Build history of the part. All positions in model axes, mm. Coordinates: 2 decimals unless noted, no trailing zeros. Order: outer loops, then holes, each group sorted by start corner. A loop starts at its lowest first (then second) coordinate and runs counter-clockwise, first axis right, second up. Notation, with made-up numbers: (-14, 77) - (27, 77) arc R11 ccw to (27, 88) - close; hole circle Ø2 at (79.25, 51). An arc over 180 degrees is marked (long way). One line per item, written item: value.
Autodesk Inventor part; units mm, degrees
ref_plane "YZ Plane" through (0, 0, 0) normal (1, 0, 0) x (0, 1, 0)
ref_plane "XZ Plane" through (0, 0, 0) normal (0, 1, 0) x (-1, 0, 0)
ref_plane "XY Plane" through (0, 0, 0) normal (0, 0, 1) x (1, 0, 0)
sketch "Sketch1" plane through (0, 0, 0) normal (0, 0, 1) x (1, 0, 0)
  line L0 (568, 44.5) -> (0, 44.5)
  line L1 (68, 0) -> (78, 15)
  line L2 (78, 15) -> (490, 15)
  line L3 (490, 15) -> (500, 0)
  line L4 (0, 0) -> (68, 0)
  line L5 (500, 0) -> (568, 0)
  line L6 (0, 30) -> (68, 30)
  line L7 (68, 30) -> (68, 23.5)
  line L8 (68, 23.5) -> (0, 23.5)
  line L9 (0, 44.5) -> (0, 30)
  line L10 (0, 23.5) -> (0, 0)
  line L11 (568, 30) -> (500, 30)
  line L12 (500, 30) -> (500, 23.5)
  line L13 (500, 23.5) -> (568, 23.5)
  line L14 (568, 0) -> (568, 23.5)
  line L15 (568, 30) -> (568, 44.5)
  dimension "d3" = 6.5
  dimension "d4" = 68
  dimension "d5" = 68
  dimension "d6" = 568
  dimension "d7" = 15
  dimension "d8" = 23.5
  dimension "d9" = 14.5
  dimension "d12" = 10
  dimension "d13" = 10
  dimension "d14" = 10
  dimension "d15" = 10
extrude "Extrusion1" add sketch "Sketch1" along normal blind 6.5
sketch "Sketch2" plane through (0, 0, 6.5) normal (0, 0, 1) x (1, 0, 0)
  line L0 (0, 0) -> (68, 0)
  line L1 (500, 0) -> (568, 0)
  line L2 (568, 0) -> (568, 23.5)
  line L3 (568, 30) -> (568, 44.5)
  line L4 (568, 44.5) -> (0, 44.5)
  line L5 (0, 44.5) -> (0, 30)
  line L6 (0, 23.5) -> (0, 0)
  line L7 (24, 0) -> (35, 0)
  line L8 (35, 0) -> (35, 9)
  line L9 (35, 9) -> (24, 9)
  line L10 (24, 9) -> (24, 0)
  circle A0 centre (42.5, 4.5) radius 2.25
  circle A1 centre (52.5, 3.901) radius 2.75
  circle A2 centre (62.5, 4.5) radius 2.25
  line L11 (544, 0) -> (533, 0)
  line L12 (533, 0) -> (533, 9)
  line L13 (533, 9) -> (544, 9)
  line L14 (544, 9) -> (544, 0)
  circle A3 centre (505.5, 4.5) radius 2.25
  circle A4 centre (515.5, 3.901) radius 2.75
  circle A5 centre (525.5, 4.5) radius 2.25
  line L15 (82.5, 44.5) -> (92.5, 44.5)
  line L16 (92.5, 44.5) -> (92.5, 40.5)
  line L17 (91.5, 39.5) -> (83.5, 39.5)
  line L18 (82.5, 40.5) -> (82.5, 44.5)
  line L19 (475.5, 44.5) -> (485.5, 44.5)
  line L20 (485.5, 44.5) -> (485.5, 40.5)
  line L21 (484.5, 39.5) -> (476.5, 39.5)
  line L22 (475.5, 40.5) -> (475.5, 44.5)
  arc A6 (82.5, 40.5) -> (83.5, 39.5) centre (83.5, 40.5) ccw
  arc A7 (91.5, 39.5) -> (92.5, 40.5) centre (91.5, 40.5) ccw
  arc A8 (475.5, 40.5) -> (476.5, 39.5) centre (476.5, 40.5) ccw
  arc A9 (484.5, 39.5) -> (485.5, 40.5) centre (484.5, 40.5) ccw
  circle A10 centre (29.5, 3.901) radius 7.5 construction
  point P0 (538.5, 9)
  point P1 (35, 4.5)
  point P2 (87.5, 39.5)
  point P3 (480.5, 39.5)
  dimension "d16" = 11
  dimension "d18" = 4.5
  dimension "d19" = 5.5
  dimension "d20" = 11
  dimension "d21" = 1
  dimension "d22" = 10
  dimension "d23" = 10
  dimension "d27" = 24
  dimension "d29" = 23
  dimension "d30" = 24
  dimension "d31" = 10
  dimension "d32" = 10
  dimension "d33" = 10
  dimension "d34" = 10
  dimension "d35" = 9
  dimension "d38" = 15
  dimension "d39" = 23
  dimension "d49" = 87.5
  dimension "d50" = 87.5
  dimension "d63" = 5
extrude "Extrusion2" cut sketch "Sketch2" against normal through all
chamfer "Chamfer1" distance 2 angle 45 4 edges at (0, 44.5, 3.25) (0, 0, 3.25) (568, 44.5, 3.25) (568, 0, 3.25)
sketch "Sketch3" plane through (0, 0, 6.5) normal (0, 0, 1) x (1, 0, 0)
  line L0 (568, 2) -> (568, 23.5)
  line L1 (0, 23.5) -> (0, 2)
  circle A0 centre (52.5, 3.901) radius 2.75
  circle A1 centre (10, 3.901) radius 2
  circle A2 centre (558, 3.901) radius 2
  point P0 (0, 0)
  dimension "d43" = 4
  dimension "d44" = 10
  dimension "d45" = 4
  dimension "d46" = 10
extrude "Extrusion3" cut sketch "Sketch3" against normal through all contours A1 | A2
sketch "Sketch4" plane through (0, 0, 6.5) normal (0, 0, 1) x (1, 0, 0)
  line L0 (568, 2) -> (568, 23.5)
  line L1 (0, 23.5) -> (0, 2)
  line L2 (2, 0) -> (24, 0)
  line L3 (35, 0) -> (68, 0)
  line L4 (500, 0) -> (533, 0)
  line L5 (544, 0) -> (566, 0)
  line L6 (10, 0) -> (18, 0)
  line L7 (18, 0) -> (18, -5)
  line L8 (16, -7) -> (12, -7)
  line L9 (10, -5) -> (10, 0)
  line L10 (48.5, 0) -> (56.5, 0)
  line L11 (56.5, 0) -> (56.5, -5)
  line L12 (54.5, -7) -> (50.5, -7)
  line L13 (48.5, -5) -> (48.5, 0)
  line L14 (511.5, 0) -> (519.5, 0)
  line L15 (519.5, 0) -> (519.5, -5)
  line L16 (517.5, -7) -> (513.5, -7)
  line L17 (511.5, -5) -> (511.5, 0)
  line L18 (550, 0) -> (558, 0)
  line L19 (558, 0) -> (558, -5)
  line L20 (556, -7) -> (552, -7)
  line L21 (550, -5) -> (550, 0)
  arc A0 (10, -5) -> (12, -7) centre (12, -5) ccw
  arc A1 (16, -7) -> (18, -5) centre (16, -5) ccw
  arc A2 (48.5, -5) -> (50.5, -7) centre (50.5, -5) ccw
  arc A3 (54.5, -7) -> (56.5, -5) centre (54.5, -5) ccw
  arc A4 (511.5, -5) -> (513.5, -7) centre (513.5, -5) ccw
  arc A5 (517.5, -7) -> (519.5, -5) centre (517.5, -5) ccw
  arc A6 (550, -5) -> (552, -7) centre (552, -5) ccw
  arc A7 (556, -7) -> (558, -5) centre (556, -5) ccw
  point P0 (0, 0)
  dimension "d51" = 2
  dimension "d52" = 8
  dimension "d53" = 8
  dimension "d54" = 8
  dimension "d55" = 8
  dimension "d56" = 7
  dimension "d57" = 10
  dimension "d58" = 30.5
  dimension "d59" = 10
  dimension "d60" = 30.5
extrude "Extrusion4" add sketch "Sketch4" against normal blind 6.5
equation "\"d5\" = d4"
equation "\"d20\" = d16"
equation "\"d23\" = d22"
equation "\"d30\" = d27"
equation "\"d45\" = d43"
equation "\"d46\" = d44"
equation "\"d59\" = d57"
equation "\"d60\" = d58"
properties part number "x_axis_chain_holder"
1. Band-saw the part on B-B, the plane z = 2.75. Count the separate pieces of the cut face and the enclosed holes in it, and give its area (3 significant figures).
Values found:
separate pieces: 1
enclosed holes: 8
area: 17,800 mm2
2. Two-plate mould, pull along X, no slides. Class faces 1 (the face through (494.93, 7.605, 3.204)), 2 (the face through (72.93, 7.395, 3.204)), 3 (the face through (280, 31, 0)): pulls with the +X half, pulls with the -X half, needs draft (parallel to the pull), parting line crosses it, or undercut.
Values found:
face 1: undercut
face 2: undercut
face 3: needs draft
3. Probe line 1 along Y through (x, z) = (505.5, 4.5); line 2 along X through (y, z) = (-3, 6); line 3 along Y through (x, z) = (47, 4). List the from-to ranges inside material, lowest first.
Values found:
line 1: y = 0 to 2.25, 6.75 to 23.5, 30 to 44.5
line 2: x = 10 to 18, 48.5 to 56.5, 511.5 to 519.5, 550 to 558
line 3: y = 0 to 23.5, 30 to 44.5
4. Band-saw the part on A-A, the plane x = 357. Give the cut face in (y, z).
Values found:
outline: (15, 0) - (44.5, 0) - (44.5, 6.5) - (15, 6.5) - close
5. Flat gauge pins, fed straight in: P1, Ø5, axis at x = 147, y = 22, coming from the -Z side; P2, Ø1.5, axis at x = 312, y = 13, coming from the +Z side; P3, Ø2, axis at x = 275, z = 1, coming from the -Y side; P4, Ø3, axis at x = 540, z = 2.5, coming from the -Y side. Where does each tip first touch, or does it go through?
Values found:
P1: stops at z = 0
P2: passes through
P3: stops at y = 15
P4: stops at y = 9
